Autodesk Inventor part; units mm, degrees
ref_plane "YZ Plane" through (0, 0, 0) normal (1, 0, 0) x (0, 1, 0)
ref_plane "XZ Plane" through (0, 0, 0) normal (0, 1, 0) x (-1, 0, 0)
ref_plane "XY Plane" through (0, 0, 0) normal (0, 0, 1) x (1, 0, 0)
sketch "Sketch1" plane through (0, 0, 0) normal (0, 0, 1) x (1, 0, 0)
  line L0 (-785, -32) -> (785, -32) construction
  line L1 (785, -32) -> (785, 0) construction
  line L2 (785, 0) -> (-785, 0) construction
  line L3 (-785, 0) -> (-785, -32) construction
  arc A0 (745, -32) -> (-745, -32) centre (0, -8688.2656) ccw
  arc A1 (-745, -32) -> (-747.7174, -34.6) centre (-744.7428, -34.989) ccw
  line L4 (-747.7174, -34.6) -> (-767.2314, -183.8295)
  arc A2 (747.7174, -34.6) -> (745, -32) centre (744.7428, -34.989) ccw
  line L5 (747.7174, -34.6) -> (767.2314, -183.8295)
  line L6 (0, 0) -> (0, -32) construction
  dimension "d0" = 1570
  dimension "d1" = 32
  dimension "d2" = 40
  dimension "d14" = 3
  dimension "d15" = 150.5
  dimension "d16" = 97.45
  dimension "d21" = 8688.2656
contour flange "Contour Flange1" sketch "Sketch1" thickness 3 bend radius 3 width 600 along (0, 0, 1) mid plane no both sides no wall seen from (757.4744, -109.2147, 0) lies toward (0.9915584, 0.1296609, 0) curves L5 A2 A0 A1 L4
bend "Bend1"
corner "Corner1"
sketch "Sketch2" plane through (0, 0, 0) normal (1, 0, 0) x (0, 1, 0)
  line L0 (3, 0) -> (3, 600) construction
  line L1 (0, 600) -> (-183.8295, 380.9205)
  line L2 (3, 0) -> (-29.011, 0)
  line L3 (0, 0) -> (-183.8295, 219.0795)
  line L4 (-183.8295, 0) -> (-183.8295, 600)
  line L5 (3, 600) -> (-183.8295, 600)
  line L6 (-183.8295, 0) -> (3, 0)
  line L7 (0, 0) -> (-32, 0)
  line L8 (-32, 600) -> (0, 600)
  line L9 (0, 0) -> (0, 600) construction
  point P0 (-29.011, 0)
  point P1 (0, 0)
  dimension "d20" = 40
extrude "Extrusion1" cut sketch "Sketch2" along normal through all both and the other way through all contours L2 L6 L4 L3
equation "\"d14\" = BendRadius"
equation "\"d3\" = Thickness"
equation "\"d4\" = BendReliefWidth"
equation "\"d5\" = BendReliefDepth"
equation "\"d6\" = MinimumRemnant"
equation "\"d7\" = TransitionRadius"
equation "\"d9\" = BendRadius"
equation "\"d11\" = CornerReliefSize"
equation "\"d12\" = GapSize"
equation "\"d13\" = JacobiRadiusSize"
equation "\"BendRadius\" = Thickness"
equation "\"BendReliefWidth\" = Thickness"
equation "\"BendReliefDepth\" = 0.5 * Thickness"
equation "\"CornerReliefSize\" = 4 * Thickness"
equation "\"MinimumRemnant\" = 2 * Thickness"
equation "\"TransitionRadius\" = BendRadius"
equation "\"JacobiRadiusSize\" = BendRadius"
equation "\"GapSize\" = Thickness"
equation "\"Поясница_радиус\" = d21"
properties part number "МОО 031 лист спина 2" material "Stainless Steel AISI 304"
Part model, mm, in its own coordinate system. A direction names the side the tool comes from. Give positions to 0.01 mm unless a question says otherwise; leave off trailing zeros. Loops run counter-clockwise (first coordinate to the right, second up) from the corner with the lowest first, then second, coordinate; pieces in that order, holes last. Notation, with made-up numbers: M -29.5,-1.75 L 24.5,-1.75 A16 cw 24.5,11.25 Z; hole C 65.5,6.25 d8. An arc over 180 degrees is marked long. Put each result on its own line as item: value. Start each with the question number.
1) Flat gauge pin, fed straight in: pin 1 (10 mm diameter, centred on x = -309.5, z = 448.5, fed in from -Y). Where does the tip first touch, or does it go through?
2) Saw through at A-A (y = -139.5). List the corners of the cut face in (x, z), then the cut area to 3 significant figures.
3) 3-axis set-ups, long thin cutter, end or side, ignore diameter. For faces 1 (the flat face through (554.46, -16.59, 19.77)), 2 (the flat face through (-757.338, -108.17, 378.791)): which of +Z, -Z, +X, -X, +Y, -Y reach the whole face in a straight line?
4) Saw through at C-C (x = 165). List the corners of the cut face in (y, z).
5) Pull direction X, two halves, no side cores. Call faces 3 (the cylindrical face through (-10.447, 2.994, 295.8)), 4 (the flat face through (757.338, -108.17, 378.791)), 5 (the flat face through (-558.06, -16.59, 19.77)), 6 (the flat face through (760.312, -107.781, 378.608)): +X half, -X half, draft (parallel to the pull), parting line (faces both ways), or undercut.
6) Saw through at D-D (z = 168). List the corners of the cut face in (x, y).
7) Probe probe 1 along X at (y, z) = (-83, 516.5); probe 2 along X at (y, z) = (-66, 205.5); probe 3 along Y at (x, z) = (557, 114.5). List the from-to ranges inside material, lowest first.
8) Saw through at B-B (z = 286). List the corners of the cut face in (x, y).
Numbers:
1. pin 1: y = -5.69
2. outline: M -764.46,166.25 L -761.43,166.25 L -761.43,600 L -764.46,600 Z; M 761.43,166.25 L 764.46,166.25 L 764.46,600 L 761.43,600 Z
2. area: 2,620 mm^2
3. face 1: -Z, +X, -X, -Y
3. face 2: +Z, -Z, -Y
4. outline: M -1.57,1.87 L 0,0 L 1.43,0 L 1.43,600 L -1.57,600 Z
5. face 3: parting line
5. face 4: undercut
5. face 5: draft
5. face 6: +X half
6. outline: M -764.65,-140.97 L -761.63,-140.97 L -747.72,-34.6 A3 cw -745,-32 A8688.27 cw 745,-32 A3 cw 747.72,-34.6 L 761.63,-140.97 L 764.65,-140.97 L 750.69,-34.21 A6 ccw 745.26,-29.01 A8691.27 ccw -745.26,-29.01 A6 ccw -750.69,-34.21 Z
7. probe 1: -757.07 to -754.05, 754.05 to 757.07
7. probe 2: -754.85 to -751.82, 751.82 to 754.85
7. probe 3: -17.87 to -14.87
8. outline: M -770.21,-183.44 L -767.23,-183.83 L -747.72,-34.6 A3 cw -745,-32 A8688.27 cw 745,-32 A3 cw 747.72,-34.6 L 767.23,-183.83 L 770.21,-183.44 L 750.69,-34.21 A6 ccw 745.26,-29.01 A8691.27 ccw -745.26,-29.01 A6 ccw -750.69,-34.21 Z
